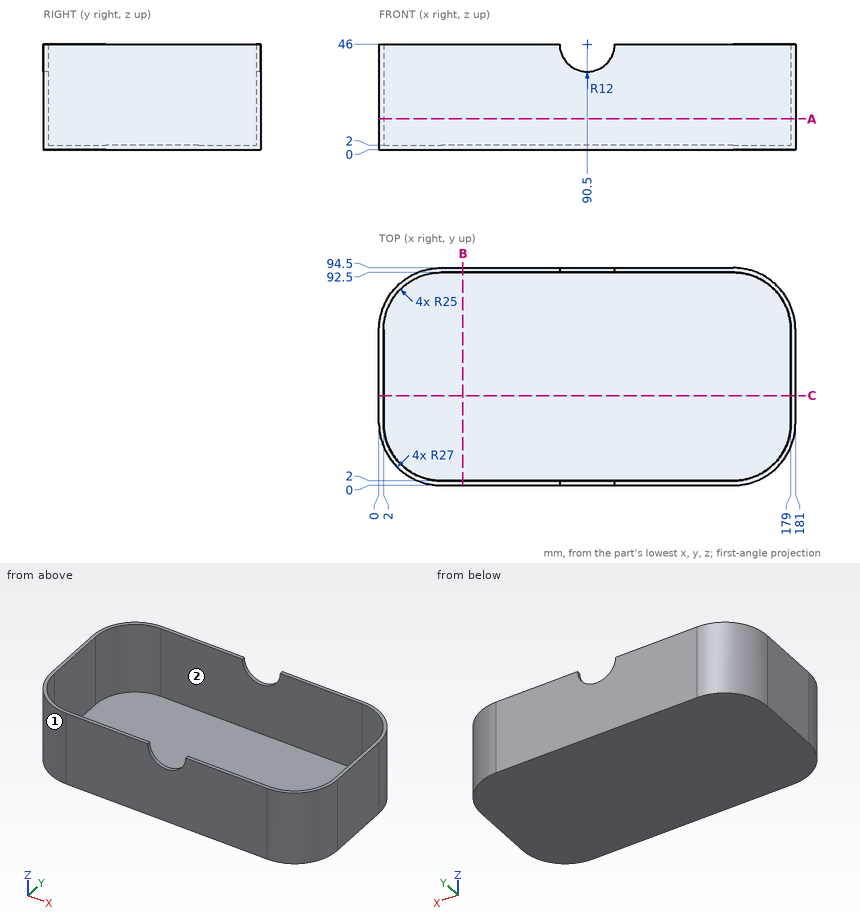
Here's the drawing with two shaded views (mm, measured from the low corner). I have some questions. A direction names the side the tool comes from. Coordinates: 2 decimals unless noted, no trailing zeros. Write each loop counter-clockwise with the first axis right and the second up, starting at its lowest first coordinate (ties: lowest second). Pieces come first, ordered by that corner, then holes.
Item 1: I want a section at C-C on y = 39. Write out the boundary of the cut face in (x, z).
Item 2: Will these pins go through, and if not, where does the flat tip stop? pin 1 (5 mm diameter, centred on x = 67, y = 22.5, fed in from +Z); pin 2 (5 mm diameter, centred on x = 87, z = 33, fed in from -Y); pin 3 (8 mm diameter, centred on y = 14, z = 30, fed in from +X).
Item 3: If I drill on line 1 (Y direction, x = 56, z = 38); line 2 (X direction, y = 34, z = 23.5); line 3 (Z direction, x = 130.5, y = 24), over which ranges is the centre line in solid material (lowest first)?
Item 4: On a 3-axis mill with a long thin cutter (end or side, diameter ignored), from which of +Z, -Z, +X, -X, +Y, -Y can I reach the whole of each face in a straight line? I mean the marked faces 1 and 2. Say none if no direction works.
Item 5: I want a section at A-A on z = 13.5. Write out the boundary of the cut face in (x, y).
Item 6: I want a section at B-B on x = 36.5. Write out the boundary of the cut face in (y, z).
Findings below:
1. outline: (0, 0) - (181, 0) - (181, 46) - (179, 46) - (179, 2) - (2, 2) - (2, 46) - (0, 46) - close
2. pin 1: stops at z = 2
2. pin 2: stops at y = 0
2. pin 3: stops at x = 179.46
3. line 1: y = 0 to 2, 92.5 to 94.5
3. line 2: x = 0 to 2, 179 to 181
3. line 3: z = 0 to 2
4. face 1: +Z, -Z, -X, -Y
4. face 2: +Z
5. outline: (0, 27) arc R27 ccw to (27, 0) - (154, 0) arc R27 ccw to (181, 27) - (181, 67.5) arc R27 ccw to (154, 94.5) - (27, 94.5) arc R27 ccw to (0, 67.5) - close; hole (2, 27) arc R25 ccw to (27, 2) - (154, 2) arc R25 ccw to (179, 27) - (179, 67.5) arc R25 ccw to (154, 92.5) - (27, 92.5) arc R25 ccw to (2, 67.5) - close
6. outline: (0, 0) - (94.5, 0) - (94.5, 46) - (92.5, 46) - (92.5, 2) - (2, 2) - (2, 46) - (0, 46) - close
